Model file for the job. Use its own axes, mm. Coordinates: 2 decimals unless noted, no trailing zeros. Loops run counter-clockwise (first coordinate to the right, second up) from the corner with the lowest first, then second, coordinate; pieces in that order, holes last.
Autodesk Inventor part; units mm, degrees
ref_plane "YZ Plane" through (0, 0, 0) normal (1, 0, 0) x (0, 1, 0)
ref_plane "XZ Plane" through (0, 0, 0) normal (0, 1, 0) x (-1, 0, 0)
ref_plane "XY Plane" through (0, 0, 0) normal (0, 0, 1) x (1, 0, 0)
sketch "Sketch1" plane through (0, 0, 0) normal (0, 0, 1) x (1, 0, 0)
  circle A0 centre (47.5, 66.25) radius 1.5
  line L0 (50.22, 62.5) -> (-50.22, 62.5) construction
  line L1 (50.22, 62.5) -> (50.22, 69.4) construction
  line L2 (50.22, 69.4) -> (-50.22, 69.4) construction
  line L3 (50.22, 69.4) -> (40.22, 69.4)
  line L4 (40.22, 69.4) -> (40.22, 62.5)
  line L5 (40.22, 62.5) -> (50.22, 62.5)
  line L6 (50.22, 62.5) -> (50.22, 69.4)
  point P0 (0, 0)
  dimension "d0" = 10
extrude "Extrusion1" add sketch "Sketch1" along normal blind 3.5
sketch "Sketch2" plane through (0, 0, 3.5) normal (0, 0, 1) x (1, 0, 0)
  circle A0 centre (47.5, 66.25) radius 1.5
  circle A1 centre (47.5, 66.25) radius 2.5
  point P0 (0, 0)
  dimension "d3" = 1
extrude "Extrusion2" cut sketch "Sketch2" against normal through all
properties part number "Screen_Spacers"
Q1. Flat gauge pin, fed straight in: P1, Ø3, axis at x = 47.5, y = 66.25, coming from the +Z side. Where does the tip first touch, or does it go through?
Answers:
P1: passes through
Q2. Drill centre lines: line 1 (Y direction, x = 47.5, z = 2.5); line 2 (Y direction, x = 49.75, z = 0.95); line 3 (X direction, y = 68, z = 0.65). Where is each one in solid material? Low to high.
Answers:
line 1: y = 62.5 to 63.75, 68.75 to 69.4
line 2: y = 62.5 to 65.16, 67.34 to 69.4
line 3: x = 40.22 to 45.71, 49.29 to 50.22
Q3. Slice it at C-C (z = 2.45). List the corners of the cut face in (x, y).
Answers:
outline: (40.22, 62.5) - (50.22, 62.5) - (50.22, 69.4) - (40.22, 69.4) - close; hole circle Ø5 at (47.5, 66.25)
Q4. Slice it at B-B (x = 47.5). List the corners of the cut face in (y, z), and give its area (3 significant figures).
Answers:
outline: (62.5, 0) - (63.75, 0) - (63.75, 3.5) - (62.5, 3.5) - close; (68.75, 0) - (69.4, 0) - (69.4, 3.5) - (68.75, 3.5) - close
area: 6.65 mm2
Q5. Mould opens along X. For faces 1 (the flat face through (40.22, 66, 2)), 2 (the flat face through (50.22, 66, 2)), 3 (the flat face through (44, 66, 0)), 4 (the cylindrical face through (49.81, 65.29, 1.77)) say: +X half, -X half, draft (parallel to the pull), parting line (faces both ways), or undercut.
Answers:
face 1: -X half
face 2: +X half
face 3: draft
face 4: undercut
Q6. Slice it at A-A (y = 66.25). List the corners of the cut face in (x, z).
Answers:
outline: (40.22, 0) - (45, 0) - (45, 3.5) - (40.22, 3.5) - close; (50, 0) - (50.22, 0) - (50.22, 3.5) - (50, 3.5) - close
